The model under review builds one solid part; all positions refer to its coordinate system, in mm. Face numbers are marked on the shaded views. A direction names the side the tool comes from. Give positions to 0.01 mm unless a question says otherwise; leave off trailing zeros. Write each loop counter-clockwise with the first axis right and the second up, starting at its lowest first coordinate (ties: lowest second). Pieces come first, ordered by that corner, then holes. Notation, with made-up numbers: M -39,28.5 L -19,28.5 A31 ccw -19,58.5 Z; hole C -6,58 d1. An arc over 180 degrees is marked long. Write item = value, one per line. Start each with the question number.
```python
from build123d import *

# Parameters (mm, degrees)
F1_DEPTH = 5
F3_DEPTH = 2
F4_R     = 1
F5_DEPTH = 25
F6_ANGLE = 180


with BuildPart() as f1:
    # F0 (on Top) → F1 (new body)
    with BuildSketch(Plane.XY):
        with BuildLine():
            ThreePointArc((-25, 14.5), (-39.5, 0), (-25, -14.5))
            Line((-25, -14.5), (25, -14.5))
            Line((25, -14.5), (25, 14.5))
            Line((25, 14.5), (-25, 14.5))
        make_face()
    extrude(amount=F1_DEPTH)

    # F2 (on face) → F3 (join)
    with BuildSketch(Plane.XY.offset(5)):
        with BuildLine():
            Line((-25, -19.5), (30, -19.5))
            Line((30, -19.5), (30, 19.5))
            Line((30, 19.5), (-25, 19.5))
            ThreePointArc((-25, 19.5), (-44.5, 0), (-25, -19.5))
        make_face()
    extrude(amount=F3_DEPTH)

    # F4 (on face) → F5 (cut)
    with BuildSketch(Plane(origin=(0, 0, 0), x_dir=(1, 0, 0), z_dir=(0, 0, -1))):
        with Locations((8.543553, 0)):
            Circle(F4_R)
        with Locations((-23.043553, 0)):
            Circle(F4_R)
    extrude(amount=-F5_DEPTH, mode=Mode.SUBTRACT)


with BuildPart() as f1_1:
    # F6: moved
    add(f1.part.rotate(Axis((30, 0, 7), (0, 1, 0)), F6_ANGLE))


with BuildPart() as f1_2:
    # F7: moved
    add(f1_1.part.moved(Location((-64.7, 0, -7))))


solid = f1_2.part
```
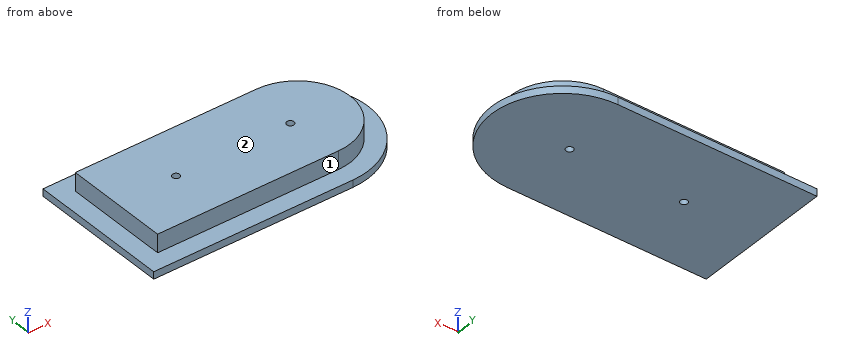
Item 1: Clearance check with flat-ended pins moving along their axes: P1, Ø1.5, axis at y = -15.5, z = 6, coming from the +X side; P2, Ø2.5, axis at x = -5.5, z = 5, coming from the -Y side; P3, Ø4, axis at x = 29, z = 4.5, coming from the +Y side; P4, Ø2.5, axis at y = 2, z = 3.5, coming from the -X side. State where each tip first meets the part, or that it passes through.
Item 2: We need section D-D, the plane x = 28. Write out the cut boundary in (y, z), and give its area (3 significant figures).
Item 3: To check wall thickness, follow probe 1 along X at (y, z) = (0, 4.5); probe 2 along X at (y, z) = (0, 0.5); probe 3 along Y at (x, z) = (15, 3.75). State the ranges of each line that lie inside material, in increasing order. Write a range as [from, to].
Item 4: We need section A-A, the plane y = 0. Write out the cut boundary in (x, z).
Item 5: We need section B-B, the plane z = 5.25. Write out the cut boundary in (x, y), and give its area (3 significant figures).
Item 6: We need section C-C, the plane y = -5.5. Write out the cut boundary in (x, z), and give its area (4 significant figures).
Item 7: For the marked faces 1 and 2, list the 3-axis set-ups (+Z, -Z, +X, -X, +Y, -Y) from which the entire face can be reached by the end or side of a thin tool; tool diameter is ignored.
Worked out:
q1.P1 = through
q1.P2 = -14.5
q1.P3 = 12.86
q1.P4 = -29.7
q2.outline = M -17.92,0 L 17.92,0 L 17.92,2 L 12.29,2 L 12.29,7 L -12.29,7 L -12.29,2 L -17.92,2 Z
q2.area = 195 mm²
q3.probe_1 = [-29.7, -14.24], [-12.24, 17.34], [19.34, 34.8]
q3.probe_2 = [-34.7, -14.24], [-12.24, 17.34], [19.34, 39.8]
q3.probe_3 = [-14.5, 14.5]
q4.outline = M -34.7,0 L -14.24,0 L -14.24,7 L -29.7,7 L -29.7,2 L -34.7,2 Z; M -12.24,0 L 17.34,0 L 17.34,7 L -12.24,7 Z; M 19.34,0 L 39.8,0 L 39.8,2 L 34.8,2 L 34.8,7 L 19.34,7 Z
q5.outline = M -29.7,-14.5 L 20.3,-14.5 A14.5 ccw 20.3,14.5 L -29.7,14.5 Z; hole C -13.24,0 d2; hole C 18.34,0 d2
q5.area = 1,770 mm²
q6.outline = M -34.7,0 L 39.01,0 L 39.01,2 L 33.72,2 L 33.72,7 L -29.7,7 L -29.7,2 L -34.7,2 Z
q6.area = 464.5 mm²
q7.face_1 = +Z, +X, -X, -Y
q7.face_2 = +Z, +X, -X, +Y, -Y
